Here's how the part is built. I have some questions about the finished solid (model axes, mm). A direction names the side the tool comes from. Coordinates: 2 decimals unless noted, no trailing zeros. Order: outer loops, then holes, each group sorted by start corner. A loop starts at its lowest first (then second) coordinate and runs counter-clockwise, first axis right, second up. Notation, with made-up numbers: (49.5, -28.75) - (89.5, -28.75) arc R17 cw to (89.5, -13.75) - close; hole circle Ø5 at (70, -37). An arc over 180 degrees is marked (long way). Answer in a Markdown table with one row per item. Add a question column.
Item 1: I want a section at D-D (y = 0.6). Count the separate pieces of the cut face and the enclosed holes in it, plus the area to 3 significant figures.
Item 2: I want a section at C-C (x = -48). Please give me the cut outline in (y, z).
Item 3: I want a section at B-B (z = -29.5). Please give me the cut outline in (x, y).
Item 4: Will this pin go through, and if not, where does the flat tip stop? pin 1 Ø2.5 at (x, z) = (-48, 13.5) entering from -Y.
Item 5: If I drill on line 1 along X through (y, z) = (1.1, -20); line 2 along X through (y, z) = (1.6, -38); line 3 along Z through (x, y) = (-16, 2.35), over which ranges is the centre line in solid material (lowest first)? Write a range as from..to.
Item 6: Thinking about a two-plate mould opening in X: for faces 3 (the cylindrical face through (56.99, 1.48, 42.65)), 4 (the cylindrical face through (-57.15, 1.48, 42.49)), 5 (the cylindrical face through (-46.42, 1.52, -37.26)), 6 (the flat face through (-1, 0, -1)), which applies, +X half, -X half, draft (parallel to the pull), parting line (faces both ways), or undercut?
Item 7: I want a section at A-A (x = -25.5). Please give me the cut outline in (y, z).
Item 8: On a 3-axis mill with a long thin cutter (end or side, diameter ignored), from which of +Z, -Z, +X, -X, +Y, -Y can I reach the whole of each face in a straight line? I mean faces 1 (the flat face through (-21, 2, -35.5)), 2 (the flat face through (1, 1, -45.5)). Say none if no direction works.
```python
from build123d import *

# Parameters (mm, degrees)
Y_KSEKLIK_EKSTR_ZYON1_DEPTH = 3
IZIM2_R                     = 1.6
KES_EKSTR_ZYON1_DEPTH       = 3
IZIM3_R                     = 1.6
KES_EKSTR_ZYON2_DEPTH       = 3
KES_EKSTR_ZYON3_DEPTH       = 3
IZIM5_R                     = 1.6
KES_EKSTR_ZYON4_DEPTH       = 3


with BuildPart() as part:
    # Çizim1 → Yükseklik-Ekstrüzyon1 (new body)
    with BuildSketch(Plane(origin=(0, 0, 0), x_dir=(1, 0, 0), z_dir=(0, 1, 0))):
        with BuildLine():
            Line((-50, -45.5), (50, -45.5))
            ThreePointArc((50, -45.5), (57.071067812, -42.571067812), (60, -35.5))
            Line((60, -35.5), (60, 35.5))
            ThreePointArc((60, 35.5), (57.071067812, 42.571067812), (50, 45.5))
            Line((50, 45.5), (-50, 45.5))
            ThreePointArc((-50, 45.5), (-57.071067812, 42.571067812), (-60, 35.5))
            Line((-60, 35.5), (-60, -35.5))
            ThreePointArc((-60, -35.5), (-57.071067812, -42.571067812), (-50, -45.5))
        make_face()
    extrude(amount=Y_KSEKLIK_EKSTR_ZYON1_DEPTH)

    # Çizim2 → Kes-Ekstrüzyon1 (cut)
    with BuildSketch(Plane(origin=(0, 3, 0), x_dir=(1, 0, 0), z_dir=(0, 1, 0))):
        with Locations(Location((50, -38, 0), (0, 0, 270))):
            Circle(IZIM2_R)
        with Locations(Location((50, 38, 0), (0, 0, 270))):
            Circle(IZIM2_R)
        with Locations(Location((-45, 38, 0), (0, 0, 270))):
            Circle(IZIM2_R)
        with Locations(Location((-45, -38, 0), (0, 0, 270))):
            Circle(IZIM2_R)
    extrude(amount=-KES_EKSTR_ZYON1_DEPTH, mode=Mode.SUBTRACT)

    # Çizim3 → Kes-Ekstrüzyon2 (cut)
    with BuildSketch(Plane(origin=(0, 3, 0), x_dir=(1, 0, 0), z_dir=(0, 1, 0))):
        with Locations(Location((45, 20, 0), (0, 0, 270))):
            Circle(IZIM3_R)
        with Locations(Location((45, -20, 0), (0, 0, 270))):
            Circle(IZIM3_R)
        with Locations(Location((5, 20, 0), (0, 0, 270))):
            Circle(IZIM3_R)
        with Locations(Location((5, -20, 0), (0, 0, 270))):
            Circle(IZIM3_R)
    extrude(amount=-KES_EKSTR_ZYON2_DEPTH, mode=Mode.SUBTRACT)

    # Çizim4 → Kes-Ekstrüzyon3 (cut)
    with BuildSketch(Plane(origin=(0, 3, 0), x_dir=(1, 0, 0), z_dir=(0, 1, 0))):
        with BuildLine():
            Line((-30, 35.5), (-12, 35.5))
            ThreePointArc((-12, 35.5), (-6, 29.5), (-12, 23.5))
            Line((-12, 23.5), (-30, 23.5))
            ThreePointArc((-30, 23.5), (-36, 29.5), (-30, 35.5))
        make_face()
    extrude(amount=-KES_EKSTR_ZYON3_DEPTH, mode=Mode.SUBTRACT)

    # Çizim5 → Kes-Ekstrüzyon4 (cut)
    with BuildSketch(Plane(origin=(0, 3, 0), x_dir=(1, 0, 0), z_dir=(0, 1, 0))):
        with Locations(Location((-48, 13.5, 0), (0, 0, 270))):
            Circle(IZIM5_R)
        with Locations(Location((-48, -13.5, 0), (0, 0, 270))):
            Circle(IZIM5_R)
    extrude(amount=-KES_EKSTR_ZYON4_DEPTH, mode=Mode.SUBTRACT)


solid = part.part
```
Values follow:
| question | item | result |
|---|---|---|
| 1 | separate pieces | 1 |
| 1 | enclosed holes | 11 |
| 1 | area | 10,400 mm^2 |
| 2 | outline | (0, -45.5) - (3, -45.5) - (3, -15.1) - (0, -15.1) - close; (0, -11.9) - (3, -11.9) - (3, 11.9) - (0, 11.9) - close; (0, 15.1) - (3, 15.1) - (3, 45.5) - (0, 45.5) - close |
| 3 | outline | (-60, 0) - (-36, 0) - (-36, 3) - (-60, 3) - close; (-6, 0) - (60, 0) - (60, 3) - (-6, 3) - close |
| 4 | pin 1 | passes through |
| 5 | line 1 | x = -60..3.4, 6.6..43.4, 46.6..60 |
| 5 | line 2 | x = -59.68..-46.6, -43.4..48.4, 51.6..59.68 |
| 5 | line 3 | z = -45.5..-35.5, -23.5..45.5 |
| 6 | face 3 | +X half |
| 6 | face 4 | -X half |
| 6 | face 5 | undercut |
| 6 | face 6 | draft |
| 7 | outline | (0, -45.5) - (3, -45.5) - (3, -35.5) - (0, -35.5) - close; (0, -23.5) - (3, -23.5) - (3, 45.5) - (0, 45.5) - close |
| 8 | face 1 | +Y, -Y |
| 8 | face 2 | -Z, +X, -X, +Y, -Y |
